Read the model definition and answer for the solid it produces. Units are mm, in the model's axes. A direction names the side the tool comes from. Coordinates: 2 decimals unless noted, no trailing zeros. Write each loop counter-clockwise with the first axis right and the second up, starting at its lowest first coordinate (ties: lowest second). Pieces come first, ordered by that corner, then holes. Notation, with made-up numbers: (45.5, -21.5) -> (69.5, -21.5) arc R12 ccw to (69.5, -11.5) -> close; hole circle Ø10 at (68, -39.5). An arc over 180 degrees is marked (long way). Return JSON: item names as keys, results as strings.
from build123d import *

# Parameters (mm, degrees)
F0_W     = 31.75
F0_H     = 11.43
F0_R     = 4.826
F1_DEPTH = 7.9375
F2_R     = 3.175
F3_DEPTH = 1.5875
F4_R     = 1.651
F5_DEPTH = 4.7625


with BuildPart() as f1:
    # F0 (on Top) → F1 (new body)
    with BuildSketch(Plane.XY):
        Rectangle(F0_W, F0_H)
        with Locations((-8.128, 0)):
            Circle(F0_R, mode=Mode.SUBTRACT)
        with Locations((8.128, 0)):
            Circle(F0_R, mode=Mode.SUBTRACT)
    extrude(amount=F1_DEPTH)

    # F2 (on face) → F3 (join)
    with BuildSketch(Plane.XY.offset(7.9375)):
        Circle(F2_R)
    extrude(amount=F3_DEPTH)

    # F4 (on face) → F5 (cut)
    with BuildSketch(Plane.XY.offset(9.525)):
        Circle(F4_R)
    extrude(amount=-F5_DEPTH, mode=Mode.SUBTRACT)


solid = f1.part
1. The part is cut by section D-D (z = 2.5). Determine the outline of the cut face in (x, y) (3 decimals), then the cut area to 3 significant figures.
Taken from the geometry:
{"outline": "(-15.875, -5.715) -> (15.875, -5.715) -> (15.875, 5.715) -> (-15.875, 5.715) -> close; hole circle Ø9.652 at (-8.128, 0); hole circle Ø9.652 at (8.128, 0)", "area": "217 mm2"}
2. The part is cut by section C-C (x = 0). Determine the outline of the cut face in (y, z) (1 decimal), then the cut area to 3 significant figures.
Taken from the geometry:
{"outline": "(-5.7, 0) -> (5.7, 0) -> (5.7, 7.9) -> (3.2, 7.9) -> (3.2, 9.5) -> (1.7, 9.5) -> (1.7, 4.8) -> (-1.7, 4.8) -> (-1.7, 9.5) -> (-3.2, 9.5) -> (-3.2, 7.9) -> (-5.7, 7.9) -> close", "area": "85.1 mm2"}
3. Consider L1, parallel to X at y = -2, z = 2 (3 decimals); L2, parallel to X at y = 0.5, z = 6.75 (3 decimals); L3, parallel to X at y = -4, z = 7.75 (3 decimals). Determine where each line is inside the solid, lowest interval first.
Taken from the geometry:
{"L1": "x = -15.875 to -12.52, -3.736 to 3.736, 12.52 to 15.875", "L2": "x = -15.875 to -12.928, -3.328 to -1.573, 1.573 to 3.328, 12.928 to 15.875", "L3": "x = -15.875 to -10.828, -5.428 to 5.428, 10.828 to 15.875"}
4. The part is cut by section B-B (y = -4). Determine the outline of the cut face in (x, z) (1 decimal).
Taken from the geometry:
{"outline": "(-15.9, 0) -> (-10.8, 0) -> (-10.8, 7.9) -> (-15.9, 7.9) -> close; (-5.4, 0) -> (5.4, 0) -> (5.4, 7.9) -> (-5.4, 7.9) -> close; (10.8, 0) -> (15.9, 0) -> (15.9, 7.9) -> (10.8, 7.9) -> close"}
5. The part is cut by section A-A (z = 5.75). Determine the outline of the cut face in (x, y) (3 decimals), then the cut area to 3 significant figures.
Taken from the geometry:
{"outline": "(-15.875, -5.715) -> (15.875, -5.715) -> (15.875, 5.715) -> (-15.875, 5.715) -> close; hole circle Ø9.652 at (-8.128, 0); hole circle Ø3.302 at (0, 0); hole circle Ø9.652 at (8.128, 0)", "area": "208 mm2"}
6. A tool of negligible diameter and unlimited length cuts with its end or side. For faces 1 (the face through (0, 0, 4.762)), 2 (the face through (0, 5.715, 4)), from which of +Z, -Z, +X, -X, +Y, -Y can it reach the whole face along a straight path? Write none if from no direction.
Taken from the geometry:
{"face 1": "+Z", "face 2": "+Z, -Z, +X, -X, +Y"}
7. Flat-ended cylindrical pins translate along their axes: pin 1 Ø3 at (x, y) = (-12, -1) entering from +Z; pin 2 Ø4 at (x, y) = (-4.5, 2) entering from +Z (3 decimals); pin 3 Ø3 at (x, y) = (0, 0) entering from +Z. Find the tip coordinate at first contact, or state that the pin passes through.
Taken from the geometry:
{"pin 1": "stops at z = 7.94", "pin 2": "stops at z = 9.525", "pin 3": "stops at z = 4.76"}
